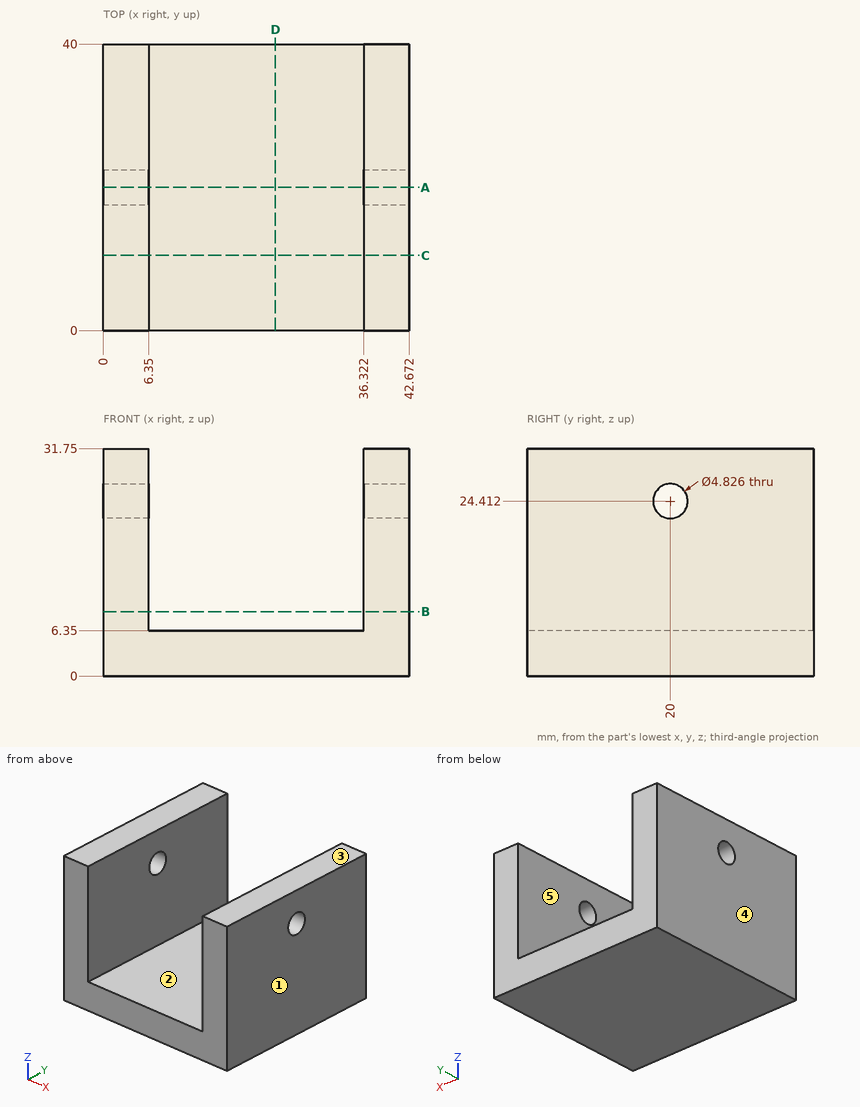
Print and shaded views of the part. All mm, measured from the part's lowest x, y and z. A direction names the side the tool comes from. Round coordinates to 2 decimals unless told otherwise and drop trailing zeros. Write each loop counter-clockwise with the first axis right and the second up, starting at its lowest first coordinate (ties: lowest second). Pieces come first, ordered by that corner, then holes. Notation, with made-up numbers: (8, -23.5) - (61, -23.5) arc R20 cw to (61, 5.5) - close; hole circle Ø1 at (-36, 0). An arc over 180 degrees is marked (long way). Write each question's results on one line, items separated by ' | '. Start each with the question number.
Item 1: Wall check: L1, parallel to X at y = 22.5, z = 22.5; L2, parallel to Z at x = 34.5, y = 13.5; L3, parallel to Y at x = 39.5, z = 23.5. Give the ranges that are in metal, low to high. Write a range as [from, to].
Item 2: Mould opens along X. For the marked faces 3, 4 and 5 say: pulls with the +X half, pulls with the -X half, needs draft (parallel to the pull), parting line crosses it, or undercut.
Item 3: Saw through at D-D (x = 24). Write the cut outline in (y, z).
Item 4: Saw through at A-A (y = 20). Write the cut outline in (x, z) (3 decimals), and give its area (3 significant figures).
Item 5: Saw through at B-B (z = 9). Write the cut outline in (x, y).
Item 6: Saw through at C-C (y = 10.5). Write the cut outline in (x, z).
Item 7: Which spindle directions (+Z, -Z, +X, -X, +Y, -Y) get a long thin tool onto all of the face, cutting with end or side? Do the marked faces 1 and 2. Say none if no direction does.
Item 8: Drop flat-ended pins along their axis: P1, Ø24, axis at x = 15, y = 18, coming from the +Z side; P2, Ø12, axis at x = 29.5, y = 29, coming from the +Z side. Give the stop position or say it passes through.
Results are:
1) L1: x = [0, 6.35], [36.32, 42.67] | L2: z = [0, 6.35] | L3: y = [0, 17.77], [22.23, 40]
2) face 3: needs draft | face 4: pulls with the -X half | face 5: undercut
3) outline: (0, 0) - (40, 0) - (40, 6.35) - (0, 6.35) - close
4) outline: (0, 0) - (42.672, 0) - (42.672, 21.999) - (36.322, 21.999) - (36.322, 6.35) - (6.35, 6.35) - (6.35, 21.999) - (0, 21.999) - close; (0, 26.825) - (6.35, 26.825) - (6.35, 31.75) - (0, 31.75) - close; (36.322, 26.825) - (42.672, 26.825) - (42.672, 31.75) - (36.322, 31.75) - close | area: 532 mm²
5) outline: (0, 0) - (6.35, 0) - (6.35, 40) - (0, 40) - close; (36.32, 0) - (42.67, 0) - (42.67, 40) - (36.32, 40) - close
6) outline: (0, 0) - (42.67, 0) - (42.67, 31.75) - (36.32, 31.75) - (36.32, 6.35) - (6.35, 6.35) - (6.35, 31.75) - (0, 31.75) - close
7) face 1: +Z, -Z, +X, +Y, -Y | face 2: +Z, +Y, -Y
8) P1: stops at z = 31.75 | P2: stops at z = 6.35
